Geometry check sheet. Reference: the model listing, model coordinates, mm. A direction names the side the tool comes from. Coordinates: 2 decimals unless noted, no trailing zeros. Write each loop counter-clockwise with the first axis right and the second up, starting at its lowest first coordinate (ties: lowest second). Pieces come first, ordered by that corner, then holes. Notation, with made-up numbers: (83.5, -21.75) - (98.5, -21.75) arc R12 ccw to (98.5, -17.75) - close; hole circle Ø6 at (82, 5.25). An arc over 180 degrees is marked (long way). Answer as a JSON object with one key per item and string values. Group by question number.
from build123d import *

# Parameters (mm, degrees)
BOSS_EXTRUDE1_DEPTH  = 14.027771651
CHAMFER1_SIZE        = 70
CHAMFER1_SIZE2       = 25.477916399
CHAMFER2_SIZE        = 70
CHAMFER2_SIZE2       = 25.477916399
REVOLVE1_ANGLE       = 180
SKETCH5_W            = 3.372425282
SKETCH5_H            = 11.999559726
CUT_EXTRUDE1_DEPTH   = 12
REVOLVE2_ANGLE       = 180
SKETCH10_W           = 9
SKETCH10_H           = 14.027771651
BOSS_EXTRUDE2_DEPTH  = 0.01
SKETCH11_W           = 1.173488445
SKETCH11_H           = 14.027771651
BOSS_EXTRUDE3_DEPTH  = 0.01
SKETCH12_W           = 3.597317039
SKETCH12_H           = 11.345384506
CUT_EXTRUDE2_DEPTH   = 12
SKETCH13_W           = 1.806847517
SKETCH13_H           = 14.027771651
BOSS_EXTRUDE4_DEPTH  = 0.01
MIRROR5_COPY_1_ANGLE = 180
MIRROR6_COPY_1_ANGLE = 180
MIRROR6_COPY_2_ANGLE = 180
SKETCH14_W           = 14.6
SKETCH14_H           = 11.534592578
CUT_EXTRUDE3_DEPTH   = 12


with BuildPart() as part:
    # Sketch1 → Boss-Extrude1 (new body)
    with BuildSketch(Plane(origin=(0, 0, 0), x_dir=(1, 0, 0), z_dir=(0, 1, 0))):
        Polygon((-28, 50), (-36, 50), (-36, -50), (-9.5, -50), (-9.5, -30), (9.5, -30), (9.5, -50), (36, -50), (36, 50), (28, 50), (28, 30), (9, 30), (9, 50), (-9, 50), (-9, 30), (-28, 30), align=None)
    extrude(amount=BOSS_EXTRUDE1_DEPTH)

    # Chamfer1
    chamfer1_edges = [part.edges().sort_by_distance(p)[0] for p in [
        (36, 7.013885825, 50),
    ]]
    chamfer1_side = [part.faces().sort_by_distance(p)[0] for p in [
        (36, 7.013885825, 0),
    ]]
    chamfer(chamfer1_edges, length=CHAMFER1_SIZE, length2=CHAMFER1_SIZE2, reference=chamfer1_side[0])

    # Chamfer2
    chamfer2_edges = [part.edges().sort_by_distance(p)[0] for p in [
        (-36, 7.013885825, 50),
    ]]
    chamfer2_side = [part.faces().sort_by_distance(p)[0] for p in [
        (-36, 7.013885825, 0),
    ]]
    chamfer(chamfer2_edges, length=CHAMFER2_SIZE, length2=CHAMFER2_SIZE2, reference=chamfer2_side[0])

    # Sketch4 → Revolve1 (revolve)
    with BuildSketch(Plane(origin=(-9.5, 0, 0), x_dir=(0, 0, -1), z_dir=(1, 0, 0))):
        with BuildLine():
            Line((-49.075, 7), (-38.925, 7))
            ThreePointArc((-38.925, 7), (-44, 12.075), (-49.075, 7))
        make_face()
    revolve1 = revolve(axis=Axis((-9.5, 7, 49.075), (0, 0, -1)), revolution_arc=REVOLVE1_ANGLE)

    # Sketch5 → Cut-Extrude1 (cut)
    with BuildSketch(Plane.XY.offset(50)):
        with Locations((-5.613787359, 7.519250292)):
            Rectangle(SKETCH5_W, SKETCH5_H)
    extrude(amount=-CUT_EXTRUDE1_DEPTH, mode=Mode.SUBTRACT)

    # Sketch8 → Revolve2 (revolve)
    with BuildSketch(Plane(origin=(-28, 0, 0), x_dir=(0, 0, -1), z_dir=(1, 0, 0))):
        with BuildLine():
            Line((38.925, 7), (49.075, 7))
            ThreePointArc((49.075, 7), (44, 12.075), (38.925, 7))
        make_face()
    revolve2 = revolve(axis=Axis((-28, 7, -38.925), (0, 0, -1)), revolution_arc=REVOLVE2_ANGLE)

    # Sketch10 → Boss-Extrude2 (add)
    with BuildSketch(Plane(origin=(0, 0, -50), x_dir=(-1, 0, 0), z_dir=(0, 0, -1))):
        with Locations((-4.5, 7.013885826)):
            Rectangle(SKETCH10_W, SKETCH10_H)
    extrude(amount=BOSS_EXTRUDE2_DEPTH)

    # Mirror2: Revolve2 across plane
    add(revolve2.mirror(Plane(origin=(0, 14.027771651, -50.01), x_dir=(0, 0, 1), z_dir=(1, 0, 0))))

    # Sketch11 → Boss-Extrude3 (add)
    with BuildSketch(Plane.XY.offset(30)):
        with Locations((0.586744223, 7.013885826)):
            Rectangle(SKETCH11_W, SKETCH11_H)
    extrude(amount=BOSS_EXTRUDE3_DEPTH)

    # Mirror4: Revolve1 across plane
    add(revolve1.mirror(Plane(origin=(0, 0, 30.01), x_dir=(0, 0, 1), z_dir=(1, 0, 0))))

    # Sketch12 → Cut-Extrude2 (cut)
    with BuildSketch(Plane.XY.offset(50)):
        with Locations((5.501341481, 7.065203355)):
            Rectangle(SKETCH12_W, SKETCH12_H)
    extrude(amount=-CUT_EXTRUDE2_DEPTH, mode=Mode.SUBTRACT)

    # Sketch13 → Boss-Extrude4 (add)
    with BuildSketch(Plane(origin=(0, 0, -30), x_dir=(-1, 0, 0), z_dir=(0, 0, -1))):
        with Locations((-17.596576242, 7.013885826)):
            Rectangle(SKETCH13_W, SKETCH13_H)
    extrude(amount=BOSS_EXTRUDE4_DEPTH)

    # Mirror5 copy 1 sketch → Mirror5 copy 1 (revolve)
    with BuildSketch(Plane(origin=(9, 0, 0), x_dir=(0, 0, -1), z_dir=(1, 0, 0))):
        with BuildLine():
            Line((38.925, 7), (49.075, 7))
            ThreePointArc((49.075, 7), (44, 12.075), (38.925, 7))
        make_face()
    revolve(axis=Axis((9, 7, -38.925), (0, 0, -1)), revolution_arc=MIRROR5_COPY_1_ANGLE)

    # Mirror6 copy 1 sketch → Mirror6 copy 1 (revolve)
    with BuildSketch(Plane(origin=(-9, 0, 0), x_dir=(0, 0, -1), z_dir=(-1, 0, 0))):
        with BuildLine():
            Line((38.925, -7), (49.075, -7))
            ThreePointArc((49.075, -7), (44, -12.075), (38.925, -7))
        make_face()
    revolve(axis=Axis((-9, 7, -38.925), (0, 0, 1)), revolution_arc=MIRROR6_COPY_1_ANGLE)

    # Mirror6 copy 2 sketch → Mirror6 copy 2 (revolve)
    with BuildSketch(Plane(origin=(28, 0, 0), x_dir=(0, 0, -1), z_dir=(-1, 0, 0))):
        with BuildLine():
            Line((38.925, -7), (49.075, -7))
            ThreePointArc((49.075, -7), (44, -12.075), (38.925, -7))
        make_face()
    revolve(axis=Axis((28, 7, -38.925), (0, 0, 1)), revolution_arc=MIRROR6_COPY_2_ANGLE)

    # Sketch14 → Cut-Extrude3 (cut)
    with BuildSketch(Plane(origin=(0, 0, -50), x_dir=(-1, 0, 0), z_dir=(0, 0, -1))):
        with Locations((-18.5, 6.982775721)):
            Rectangle(SKETCH14_W, SKETCH14_H)
        with Locations((18.5, 6.982775721)):
            Rectangle(SKETCH14_W, SKETCH14_H)
    extrude(amount=-CUT_EXTRUDE3_DEPTH, mode=Mode.SUBTRACT)


solid = part.part
(1) Section check B-B (x = 13). Record the cut outline in (y, z), and give its area (3 significant figures).
(2) Material ranges on L1, parallel to Z at x = 2, y = 10.5; L2, parallel to X at y = 3, z = 44; L3, parallel to X at y = 4.75, z = 45.5, recorded low to high. Write a range as [from, to].
(3) Draft check along Z on faces 5 (the face through (9, 7, -38)), 6 (the face through (-23.083, 6.916, 15.49)), 7 (the face through (-4, 7, -50)). Enter one of: +Z half, -Z half, draft (parallel to the pull), parting line (faces both ways), or undercut.
(4) Set-up check for faces 1 (the face through (1, 0, -10)), 2 (the face through (-25.8, 7, -44)), 3 (the face through (-9.5, 7, 38)), 4 (the face through (-18, 7, -30)): record each of +Z, -Z, +X, -X, +Y, -Y from which the full face is reachable in a straight line by a thin tool's end or side.
(5) Section check A-A (z = -33). Record the cut outline in (x, y).
(6) Gauge pin test, flat ends, axial feed: pin 1 (8 mm diameter, centred on y = 4, z = 25, fed in from -X); pin 2 (6 mm diameter, centred on y = 5.5, z = -9.5, fed in from -X); pin 3 (1.3 mm diameter, centred on x = 0.5, y = 9, fed in from +Z). Record the tip position at first contact, or that the pin passes through.
(7) Section check C-C (z = 14). Record the cut outline in (x, y).
Conclusion:
{
 "1": {"outline": "(0, -30) - (14.03, -30) - (14.03, 43.19) - (0, 43.19) - close", "area": "1,030 mm^2"},
 "2": {"L1": "z = [-50.01, 30]", "L2": "x = [-12.71, -7.3], [7.3, 12.71]", "L3": "x = [-12.16, -7.3], [7.3, 12.16]"},
 "3": {"face 5": "undercut", "face 6": "+Z half", "face 7": "-Z half"},
 "4": {"face 1": "+Z, -Z, +X, -X, -Y", "face 2": "-Z, +Y, -Y", "face 3": "none", "face 4": "+Y, -Y"},
 "5": {"outline": "(-36, 0) - (-28, 0) - (-28, 14.03) - (-36, 14.03) - close; (-9, 0) - (9, 0) - (9, 14.03) - (-9, 14.03) - close; (28, 0) - (36, 0) - (36, 14.03) - (28, 14.03) - close"},
 "6": {"pin 1": "stops at x = -21.08", "pin 2": "stops at x = -33.27", "pin 3": "stops at z = 30.01"},
 "7": {"outline": "(-23.63, 0) - (23.63, 0) - (23.63, 14.03) - (-23.63, 14.03) - close"}
}
